Here's how the part is built. I have some questions about the finished solid (model axes, mm). Coordinates: 2 decimals unless noted, no trailing zeros. Loops run counter-clockwise (first coordinate to the right, second up) from the corner with the lowest first, then second, coordinate; pieces in that order, holes last. Notation, with made-up numbers: M 28,-16 L 74,-16 A30 ccw 74,14 Z; hole C 39.5,47 d10. An arc over 180 degrees is marked long. Use one line per item in the form item = value. Start each with the question number.
(1) Imagine slicing it at A-A, the plane z = 12.7. Please give me the cut outline in (x, y) (3 decimals).
(2) Imagine slicing it at C-C, the plane y = 1.5. Please give me the cut outline in (x, z) (3 decimals).
(3) Thinking about a two-plate mould opening in X: for faces 1 (the cylindrical face through (-2.06, 0.09, 3.4)), 2 (the flat face through (-63.5, 0, -1)), 3 (the flat face through (-1, 0, 63.5)), which applies, +X half, -X half, draft (parallel to the pull), parting line (faces both ways), or undercut?
(4) Imagine slicing it at B-B, the plane x = 0. Please give me the cut outline in (y, z) (3 decimals), and give its area (3 significant figures).
(5) Please list where these lines run through material, in increasing order: L1, parallel to X at y = -2.5, z = 12; L2, parallel to Z at x = 0, y = 0.75 (3 decimals); L3, parallel to X at y = -2.5, z = 21.5.
(6) Will this pin go through, and if not, where does the flat tip stop? P1, Ø17, axis at x = 0, z = 12.7, coming from the -Y side.
```python
from build123d import *

# Parameters (mm, degrees)
F0_W     = 127
F0_H     = 127
F0_R     = 9.525
F1_DEPTH = 6.35


with BuildPart() as f1:
    # F0 (on Front) → F1 (new body, symmetric)
    with BuildSketch(Plane.XZ):
        Rectangle(F0_W, F0_H)
        with Locations((0, 12.7)):
            Circle(F0_R, mode=Mode.SUBTRACT)
    extrude(amount=F1_DEPTH, both=True)


solid = f1.part
```
Answer:
q1.outline = M -63.5,-6.35 L -9.525,-6.35 L -9.525,6.35 L -63.5,6.35 Z; M 9.525,-6.35 L 63.5,-6.35 L 63.5,6.35 L 9.525,6.35 Z
q2.outline = M -63.5,-63.5 L 63.5,-63.5 L 63.5,63.5 L -63.5,63.5 Z; hole C 0,12.7 d19.05
q3.face_1 = undercut
q3.face_2 = -X half
q3.face_3 = draft
q4.outline = M -6.35,-63.5 L 6.35,-63.5 L 6.35,3.175 L -6.35,3.175 Z; M -6.35,22.225 L 6.35,22.225 L 6.35,63.5 L -6.35,63.5 Z
q4.area = 1,370 mm²
q5.L1 = -63.5 to -9.5, 9.5 to 63.5
q5.L2 = -63.5 to 3.175, 22.225 to 63.5
q5.L3 = -63.5 to -3.64, 3.64 to 63.5
q6.P1 = through
